```python
from build123d import *

# Parameters (mm, degrees)
ESBO_O1_R                = 2.4
RESSALTO_EXTRUS_O1_DEPTH = 6
ESBO_O2_W                = 63.7
ESBO_O2_H                = 61
RESSALTO_EXTRUS_O2_DEPTH = 14.8
CHANFRO1_SIZE            = 1
ESBO_O3_R                = 6.25
CORTE_EXTRUS_O1_DEPTH    = 16.8
FILETE1_R                = 4.65
RESSALTO_EXTRUS_O4_DEPTH = 13.3
RESSALTO_EXTRUS_O5_START = -2.2
RESSALTO_EXTRUS_O5_DEPTH = 2.2
RESSALTO_EXTRUS_O6_START = 2.2
RESSALTO_EXTRUS_O6_DEPTH = 2.2
RESSALTO_EXTRUS_O7_START = 3.5
ESBO_O7_R                = 9.3
ESBO_O7_R_2              = 6.25
RESSALTO_EXTRUS_O7_DEPTH = 3.5


with BuildPart() as part:
    # Esboço1 → Ressalto-extrusão1 (new body)
    with BuildSketch(Plane(origin=(0, 0, 0), x_dir=(1, 0, 0), z_dir=(0, 1, 0))):
        Polygon((-41.15, -1.7), (-31.85, -1.7), (-31.85, 30.5), (41.15, 30.5), (41.15, 1.7), (31.85, 1.7), (31.85, -30.5), (-41.15, -30.5), align=None)
        with Locations(Location((-36.5, -8.7, 0), (0, 0, 270))):
            Circle(ESBO_O1_R, mode=Mode.SUBTRACT)
        with Locations(Location((-36.5, -23.5, 0), (0, 0, 270))):
            Circle(ESBO_O1_R, mode=Mode.SUBTRACT)
        with Locations(Location((36.5, 8.7, 0), (0, 0, 270))):
            Circle(ESBO_O1_R, mode=Mode.SUBTRACT)
        with Locations(Location((36.5, 23.5, 0), (0, 0, 270))):
            Circle(ESBO_O1_R, mode=Mode.SUBTRACT)
    extrude(amount=RESSALTO_EXTRUS_O1_DEPTH)

    # Esboço2 → Ressalto-extrusão2 (add)
    with BuildSketch(Plane(origin=(0, 6, 0), x_dir=(1, 0, 0), z_dir=(0, 1, 0))):
        Rectangle(ESBO_O2_W, ESBO_O2_H)
    extrude(amount=RESSALTO_EXTRUS_O2_DEPTH)

    # Chanfro1
    chanfro1_edges = [part.edges().sort_by_distance(p)[0] for p in [
        (31.85, 10.4, 30.5),
        (-31.85, 10.4, -30.5),
        (0, 20.8, -30.5),
        (31.85, 13.4, -30.5),
        (31.85, 20.8, 0),
        (0, 20.8, 30.5),
        (-31.85, 13.4, 30.5),
        (-31.85, 20.8, 0),
    ]]
    chamfer(chanfro1_edges, length=CHANFRO1_SIZE)

    # Esboço3 → Corte-extrusão1 (cut)
    with BuildSketch(Plane(origin=(0, 20.8, 0), x_dir=(1, 0, 0), z_dir=(0, 1, 0))):
        with Locations(Location((0, 0, 0), (0, 0, 270))):
            Circle(ESBO_O3_R)
    extrude(amount=-CORTE_EXTRUS_O1_DEPTH, mode=Mode.SUBTRACT)

    # Filete1
    filete1_edges = [part.edges().sort_by_distance(p)[0] for p in [
        (41.15, 3, -30.5),
        (41.15, 3, -1.7),
        (31.85, 3, -1.7),
        (-31.85, 3, 1.7),
        (-41.15, 3, 1.7),
        (-41.15, 3, 30.5),
    ]]
    fillet(filete1_edges, radius=FILETE1_R - 0.0001)  # a hair under: the kernel refuses the full size

    # Esboço4 → Ressalto-extrusão4 (add)
    with BuildSketch(Plane(origin=(0, 0, -29.5), x_dir=(-1, 0, 0), z_dir=(0, 0, -1))):
        with BuildLine():
            Line((-31.85, 19.8), (-22.05, 19.8))
            Line((-22.05, 19.8), (-22.05, 28.1))
            ThreePointArc((-22.05, 28.1), (-23.213022612, 31.269384798), (-26.15, 32.934252786))
            Line((-26.15, 32.934252786), (-26.15, 30.783281573))
            ThreePointArc((-26.15, 30.783281573), (-26.95, 25.3), (-27.75, 30.783281573))
            Line((-27.75, 30.783281573), (-27.75, 32.934252786))
            ThreePointArc((-27.75, 32.934252786), (-30.686977388, 31.269384798), (-31.85, 28.1))
            Line((-31.85, 28.1), (-31.85, 19.8))
        make_face()
    extrude(amount=-RESSALTO_EXTRUS_O4_DEPTH)

    # Esboço5 → Ressalto-extrusão5 (add)
    with BuildSketch(Plane.XY.offset(-16.2).offset(RESSALTO_EXTRUS_O5_START)):
        with BuildLine():
            Line((26.15, 30.783281573), (26.15, 28.1))
            ThreePointArc((26.15, 28.1), (26.95, 27.3), (27.75, 28.1))
            Line((27.75, 28.1), (27.75, 30.783281573))
            ThreePointArc((27.75, 30.783281573), (26.95, 25.3), (26.15, 30.783281573))
        make_face()
    extrude(amount=RESSALTO_EXTRUS_O5_DEPTH)

    # Esboço6 → Ressalto-extrusão6 (add)
    with BuildSketch(Plane(origin=(0, 4, 0), x_dir=(1, 0, 0), z_dir=(0, 1, 0)).offset(RESSALTO_EXTRUS_O6_START)):
        with BuildLine():
            Line((-3.011276291, -4.300548233), (-3.584852727, -5.119700277))
            ThreePointArc((-3.584852727, -5.119700277), (0, 6.25), (3.584852727, -5.119700277))
            Line((3.584852727, -5.119700277), (3.011276291, -4.300548233))
            ThreePointArc((3.011276291, -4.300548233), (0, 5.25), (-3.011276291, -4.300548233))
        make_face()
    extrude(amount=-RESSALTO_EXTRUS_O6_DEPTH)

    # Esboço7 → Ressalto-extrusão7 (add)
    with BuildSketch(Plane(origin=(0, 20.8, 0), x_dir=(1, 0, 0), z_dir=(0, 1, 0)).offset(RESSALTO_EXTRUS_O7_START)):
        with Locations(Location((0, 0, 0), (0, 0, 90))):
            Circle(ESBO_O7_R)
        with Locations(Location((0, 0, 0), (0, 0, 270))):
            Circle(ESBO_O7_R_2, mode=Mode.SUBTRACT)
    extrude(amount=-RESSALTO_EXTRUS_O7_DEPTH)


solid = part.part
```
The model under review builds one solid part; all positions refer to its coordinate system, in mm. A direction names the side the tool comes from. Give positions to 0.01 mm unless a question says otherwise; leave off trailing zeros. Write each loop counter-clockwise with the first axis right and the second up, starting at its lowest first coordinate (ties: lowest second). Pieces come first, ordered by that corner, then holes.
(1) Tool access review of faces 4 (the flat face through (31.85, 11, 0)), 5 (the flat face through (2, 10, -30.5)), 6 (the flat face through (0, 4, 0)), 7 (the flat face through (22.05, 24, -23)): name each direction out of +Z, -Z, +X, -X, +Y, -Y from which nothing blocks a thin tool from reaching the whole face with its end or side.
(2) Consider section D-D, the plane z = 14.5. Give the boundary of the cut face in (x, y), and give its area (3 significant figures).
(3) To check wall thickness, follow L1, parallel to X at y = 4.35, z = -8.7; L2, parallel to Z at x = 0, y = 19.25; L3, parallel to X at y = 3.5, z = 6. State the ranges of each line that lie inside material, in increasing order.
(4) For P1, Ø8, axis at y = 25, z = -22, coming from the -X side; P2, Ø4.5, axis at x = -36.5, z = 8.7, coming from the +Y side; P3, Ø10, axis at x = 0, z = 0, coming from the +Y side; P4, Ø4, axis at x = 8.5, y = 25, coming from the -Z side, all flat-tipped, find the tip position at first contact; note any pin that passes through.
(5) The part is to be moulded in two halves that separate along Z. For faces 1 (the flat face through (-2.2, 24.3, -6.1)), 2 (the cylindrical face through (34.157, 2.958, -9.22)), 3 (the flat face through (26, 27, -18.4)), say which applies: released by +Z, released by -Z, zero draft, split by the parting line, or undercut.
(6) Consider section C-C, the plane y = 15.5. Give the boundary of the cut face in (x, z), and give its area (3 significant figures).
(7) Consider section A-A, the plane z = 23.5. Give the boundary of the cut face in (x, y), and give its area (3 significant figures).
(8) Consider section B-B, the plane x = 0. Give the boundary of the cut face in (y, z).
Returned:
1. face 4: +Z, +X, +Y
1. face 5: -Z, +X, -X, +Y, -Y
1. face 6: +Y
1. face 7: +Z, -Z, -X, +Y
2. outline: (-41.15, 0) - (31.85, 0) - (31.85, 19.8) - (30.85, 20.8) - (-30.85, 20.8) - (-31.85, 19.8) - (-31.85, 6) - (-41.15, 6) - close
2. area: 1,380 mm2
3. L1: x = -31.85 to 34.1, 38.9 to 41.15
3. L2: z = -30.5 to -6.25, 6.25 to 30.5
3. L3: x = -41.14 to 31.85
4. P1: stops at x = 22.05
4. P2: passes through
4. P3: stops at y = 4
4. P4: stops at z = -6.53
5. face 1: zero draft
5. face 2: undercut
5. face 3: released by -Z
6. outline: (-31.85, -29.5) - (-30.85, -30.5) - (30.85, -30.5) - (31.85, -29.5) - (31.85, 29.5) - (30.85, 30.5) - (-30.85, 30.5) - (-31.85, 29.5) - close; hole circle Ø12.5 at (0, 0)
6. area: 3,760 mm2
7. outline: (-41.15, 0) - (-38.9, 0) - (-38.9, 6) - (-41.15, 6) - close; (-34.1, 0) - (31.85, 0) - (31.85, 19.8) - (30.85, 20.8) - (-30.85, 20.8) - (-31.85, 19.8) - (-31.85, 6) - (-34.1, 6) - close
7. area: 1,350 mm2
8. outline: (0, -30.5) - (19.8, -30.5) - (20.8, -29.5) - (20.8, -9.3) - (24.3, -9.3) - (24.3, -6.25) - (6.2, -6.25) - (6.2, -5.25) - (4, -5.25) - (4, 6.25) - (24.3, 6.25) - (24.3, 9.3) - (20.8, 9.3) - (20.8, 29.5) - (19.8, 30.5) - (0, 30.5) - close
